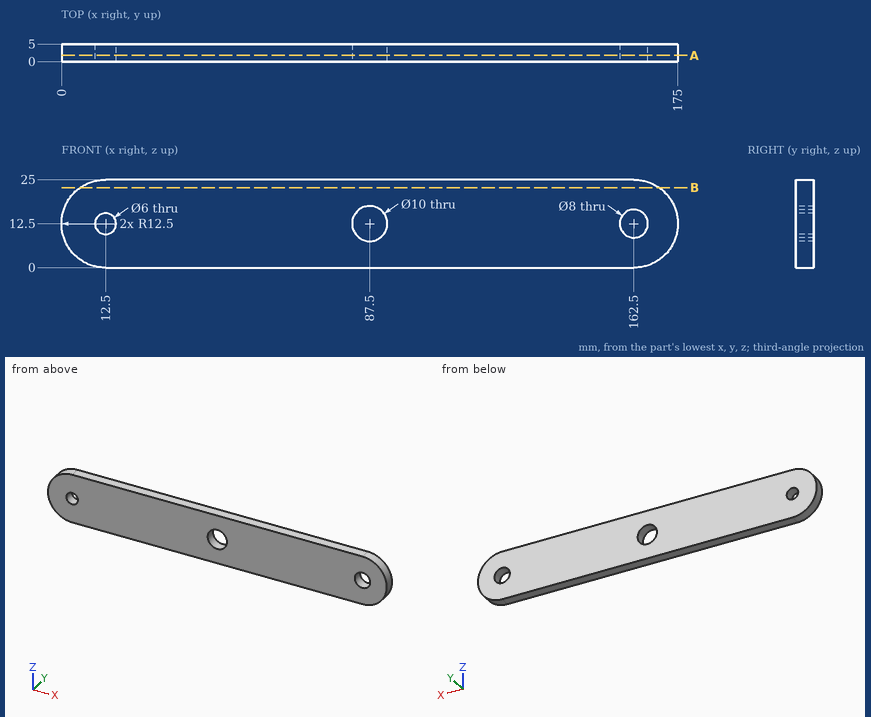
Input: dimensioned drawing with shaded views. Units: mm. Origin: part minimum x, y, z. Give positions to 0.01 mm unless a question says otherwise; leave off trailing zeros. Write each loop counter-clockwise with the first axis right and the second up, starting at its lowest first coordinate (ties: lowest second). Pieces come first, ordered by that corner, then holes. Notation, with made-up numbers: (-13, 11.5) -> (-7, 11.5) arc R22 cw to (-7, 48.5) -> close; hole circle Ø10 at (-24.75, 3). An arc over 180 degrees is marked (long way). Return JSON: item names as keys, results as strings. Group by question number.
1. Material intervals for line 1 (Z direction, x = 162, y = 3.2); line 2 (Z direction, x = 87.5, y = 2.75); line 3 (X direction, y = 3.5, z = 9), sorted ascending. Write a range as from..to.
2. Section A-A, the plane y = 1.75. Output: boundary loops of the cut face in (x, z), then the cut area to 3 significant figures.
3. Section B-B, the plane z = 22.75. Output: boundary loops of the cut face in (x, y), then the cut area to 3 significant figures.
Determined:
{
 "1": {"line 1": "z = 0..8.53, 16.47..25", "line 2": "z = 0..7.5, 17.5..25", "line 3": "x = 0.5..83.93, 91.07..160.56, 164.44..174.5"},
 "2": {"outline": "(12.5, 0) -> (162.5, 0) arc R12.5 ccw to (162.5, 25) -> (12.5, 25) arc R12.5 ccw to start; hole circle Ø6 at (12.5, 12.5); hole circle Ø10 at (87.5, 12.5); hole circle Ø8 at (162.5, 12.5)", "area": "4,080 mm2"},
 "3": {"outline": "(5.35, 0) -> (169.65, 0) -> (169.65, 5) -> (5.35, 5) -> close", "area": "822 mm2"}
}
